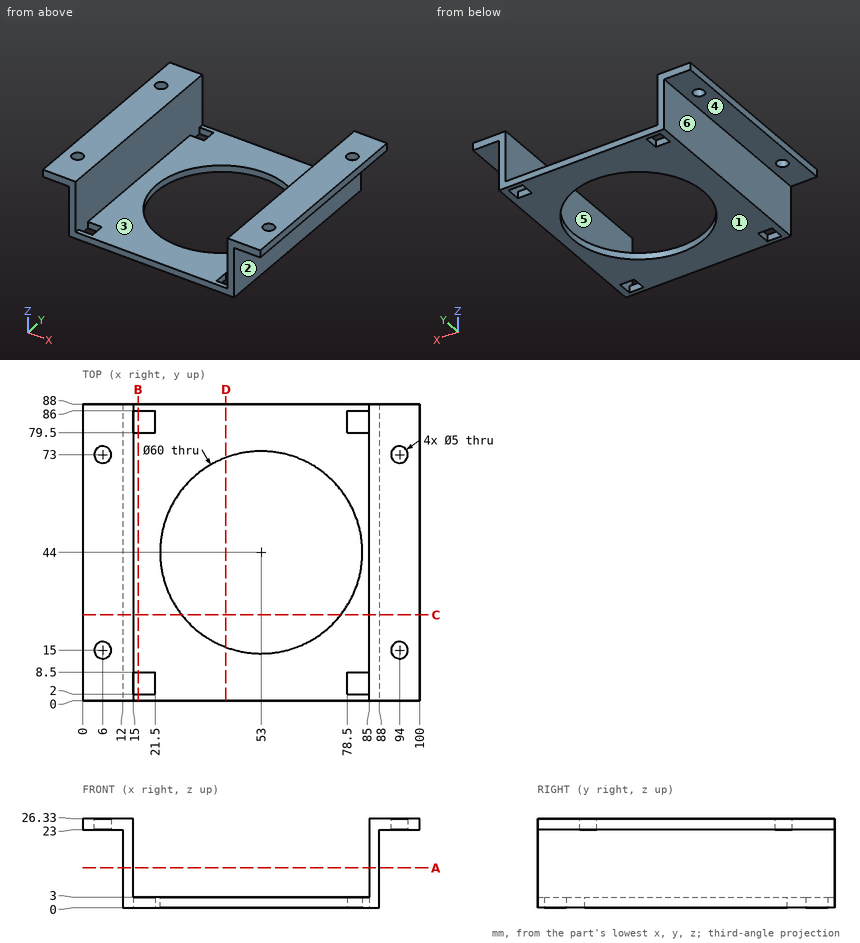
Print and shaded views of the part. All mm, measured from the part's lowest x, y and z. A direction names the side the tool comes from. Coordinates: 2 decimals unless noted, no trailing zeros. Loops run counter-clockwise (first coordinate to the right, second up) from the corner with the lowest first, then second, coordinate; pieces in that order, holes last. Notation, with made-up numbers: (-21.5, -32) -> (4.5, -32) arc R18 cw to (4.5, -12) -> close; hole circle Ø6 at (17.25, -2.5). An arc over 180 degrees is marked (long way). Use a Markdown table: item, result. Add a question column.
Item 1: Band-saw the part on A-A on z = 11.75. Write the cut outline in (x, y), plus the area to 3 significant figures.
Item 2: Flat gauge pins, fed straight in: P1, Ø12, axis at y = 20, z = 6.5, coming from the -X side; P2, Ø3, axis at y = 58.5, z = 19, coming from the +X side; P3, Ø13, axis at x = 96, y = 48.5, coming from the -Z side. Where does each tip first touch, or does it go through?
Item 3: Which spindle directions (+Z, -Z, +X, -X, +Y, -Y) get a long thin tool onto all of the face, cutting with end or side? Do the marked faces 1, 2 and 3. Say none if no direction does.
Item 4: Probe probe 1 along Y at (x, z) = (94, 25.1); probe 2 along X at (y, z) = (73, 25.15); probe 3 along X at (y, z) = (71.5, 19.75). List the from-to ranges inside material, lowest first.
Item 5: Band-saw the part on C-C on y = 25.5. Write the cut outline in (x, z).
Item 6: Band-saw the part on B-B on x = 16.5. Write the cut outline in (y, z).
Item 7: Band-saw the part on D-D on x = 42.5. Write the cut outline in (y, z).
Item 8: Pull direction X, two halves, no side cores. Call the marked faces 4, 5 and 6: +X half, -X half, draft (parallel to the pull), parting line (faces both ways), or undercut.
Geometry says:
| question | item | result |
|---|---|---|
| 1 | outline | (12, 0) -> (15, 0) -> (15, 88) -> (12, 88) -> close; (85, 0) -> (88, 0) -> (88, 88) -> (85, 88) -> close |
| 1 | area | 528 mm² |
| 2 | P1 | x = 12 |
| 2 | P2 | x = 88 |
| 2 | P3 | z = 23 |
| 3 | face 1 | -Z, +X, -X, +Y, -Y |
| 3 | face 2 | -Z, +X, +Y, -Y |
| 3 | face 3 | +Z, +Y, -Y |
| 4 | probe 1 | 0 to 12.5, 17.5 to 70.5, 75.5 to 88 |
| 4 | probe 2 | 0 to 3.5, 8.5 to 15, 85 to 91.5, 96.5 to 100 |
| 4 | probe 3 | 12 to 15, 85 to 88 |
| 5 | outline | (0, 23) -> (12, 23) -> (12, 0) -> (29.38, 0) -> (29.38, 3) -> (15, 3) -> (15, 26.33) -> (0, 26.33) -> close; (76.62, 0) -> (88, 0) -> (88, 23) -> (100, 23) -> (100, 26.33) -> (85, 26.33) -> (85, 3) -> (76.62, 3) -> close |
| 6 | outline | (0, 0) -> (2, 0) -> (2, 3) -> (0, 3) -> close; (8.5, 0) -> (79.5, 0) -> (79.5, 3) -> (8.5, 3) -> close; (86, 0) -> (88, 0) -> (88, 3) -> (86, 3) -> close |
| 7 | outline | (0, 0) -> (15.9, 0) -> (15.9, 3) -> (0, 3) -> close; (72.1, 0) -> (88, 0) -> (88, 3) -> (72.1, 3) -> close |
| 8 | face 4 | draft |
| 8 | face 5 | undercut |
| 8 | face 6 | -X half |
